Design review of the part built by this model. Coordinates are the model's own, in mm. Round coordinates to 2 decimals unless told otherwise and drop trailing zeros. Write each loop counter-clockwise with the first axis right and the second up, starting at its lowest first coordinate (ties: lowest second). Pieces come first, ordered by that corner, then holes. Notation, with made-up numbers: (47, 83.25) -> (89, 83.25) arc R27 ccw to (89, 104.25) -> close; hole circle Ø5 at (37.25, -7). An arc over 180 degrees is marked (long way). Write item = value, one per line. Start each with the question number.
Item 1: To check wall thickness, follow L1, parallel to Y at x = 34, z = 9.25; L2, parallel to Y at x = 13, z = 3.25; L3, parallel to X at y = 25.5, z = 9.75. State the ranges of each line that lie inside material, in increasing order.
Item 2: Add section C-C, the plane x = 33. State the section outline as (y, z) points.
Item 3: Add section A-A, the plane z = 2. State the section outline as (x, y) points.
Item 4: Add section B-B, the plane y = 30. State the section outline as (x, z) points, then the cut area to 3 significant figures.
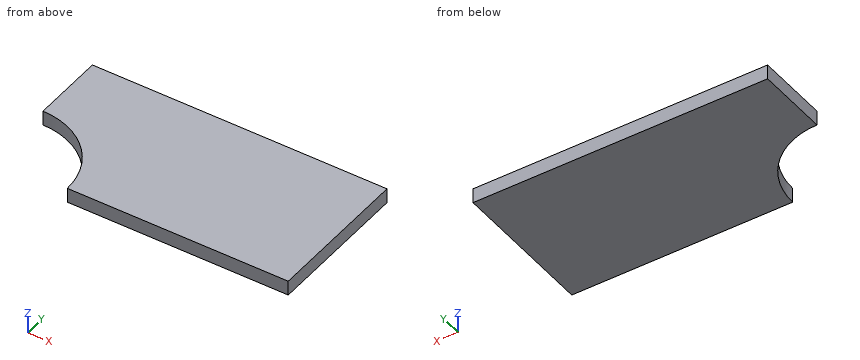
from build123d import *

# Parameters (mm, degrees)
CYLINDER_R     = 50
CYLINDER_DEPTH = 10
BOX_W          = 200
BOX_H          = 100
BOX_DEPTH      = 10


with BuildPart() as cylinder:
    # Cylinder → Cylinder (new body)
    with BuildSketch(Plane.XY):
        Circle(CYLINDER_R)
    extrude(amount=CYLINDER_DEPTH)


with BuildPart() as cut:
    # Box → Box (new body)
    with BuildSketch(Plane.XY):
        with Locations((100, 50)):
            Rectangle(BOX_W, BOX_H)
    extrude(amount=BOX_DEPTH)

    # Cut: cut Cylinder
    add(cylinder.part, mode=Mode.SUBTRACT)


solid = cut.part
Result set:
q1.L1 = 36.66 to 100
q1.L2 = 48.28 to 100
q1.L3 = 43.01 to 200
q2.outline = (37.56, 0) -> (100, 0) -> (100, 10) -> (37.56, 10) -> close
q3.outline = (0, 50) arc R50 cw to (50, 0) -> (200, 0) -> (200, 100) -> (0, 100) -> close
q4.outline = (40, 0) -> (200, 0) -> (200, 10) -> (40, 10) -> close
q4.area = 1,600 mm²
